Geometry check sheet. Reference: drawing and pictorial views, mm from the part's lowest x, y, z. A direction names the side the tool comes from. Give positions to 0.01 mm unless a question says otherwise; leave off trailing zeros. Loops run counter-clockwise (first coordinate to the right, second up) from the corner with the lowest first, then second, coordinate; pieces in that order, holes last. Notation, with made-up numbers: (68.25, 50.25) -> (115.25, 50.25) arc R15 cw to (115.25, 66.25) -> close; hole circle Ø8 at (48, 87). An arc over 180 degrees is marked (long way). Answer in a Markdown table with one row per item. Add a question column.
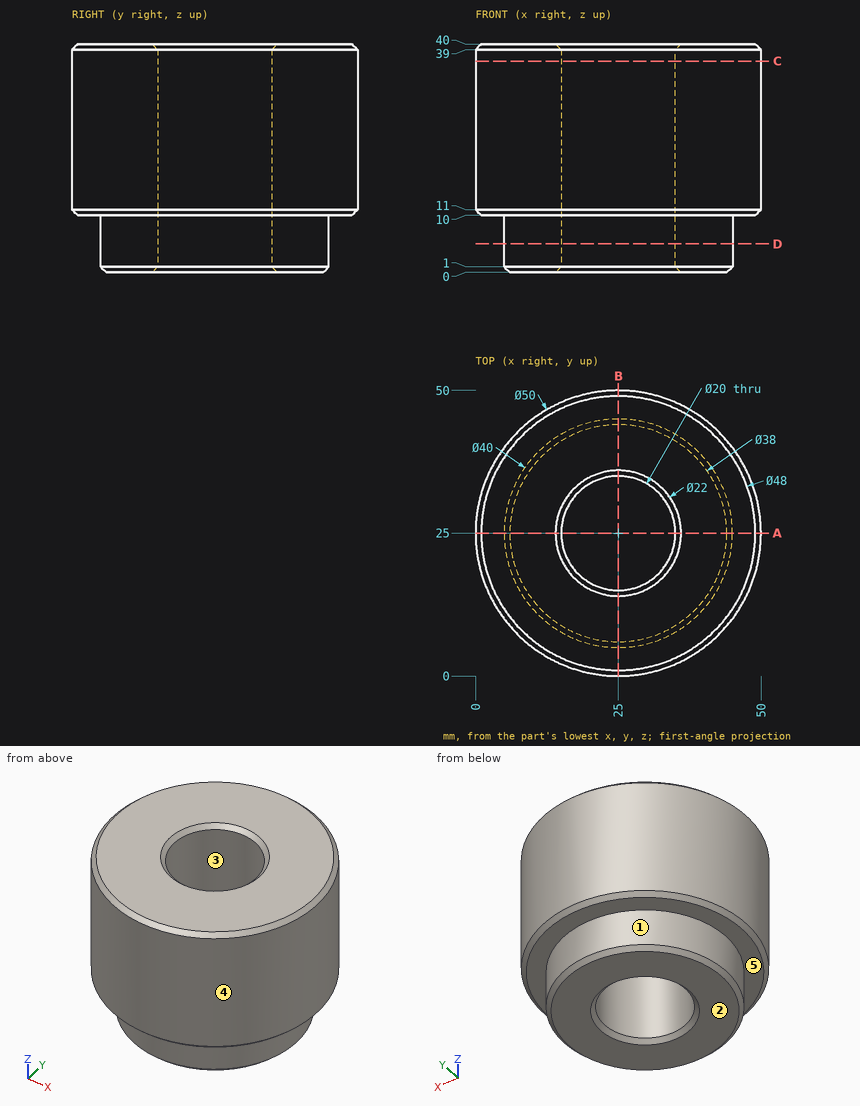
1. Release check for a two-part mould opening along Y. For the marked faces 1, 2 and 3 record: released by +Y, released by -Y, zero draft, split by the parting line, or undercut.
2. Sectioned sample at A-A (y = 25). Enter the section's corners in (x, z).
3. Sectioned sample at C-C (z = 37). Enter the section's corners in (x, y), plus the area to 3 significant figures.
4. Sectioned sample at D-D (z = 5). Enter the section's corners in (x, y), plus the area to 3 significant figures.
5. Material ranges on L1, parallel to Y at x = 25, z = 11; L2, parallel to Z at x = 42, y = 11; L3, parallel to Y at x = 17, z = 6, recorded low to high. Write a range as from..to.
6. Access from +Z, -Z, +X, -X, +Y, -Y to the whole of each face (thin tool, end or side, straight path). Record for the marked faces 4 and 5.
7. Gauge pin test, flat ends, axial feed: pin 1 Ø8 at (x, z) = (5.5, 24) entering from +Y; pin 2 Ø1.5 at (x, y) = (13.5, 42.5) entering from -Z; pin 3 Ø6 at (y, z) = (40.5, 10) entering from -X; pin 4 Ø10 at (x, y) = (27, 32) entering from +Z. Record the tip position at first contact, or that the pin passes through.
Response:
| question | item | result |
|---|---|---|
| 1 | face 1 | split by the parting line |
| 1 | face 2 | zero draft |
| 1 | face 3 | undercut |
| 2 | outline | (0, 11) -> (1, 10) -> (5, 10) -> (5, 1) -> (6, 0) -> (14, 0) -> (15, 1) -> (15, 39) -> (14, 40) -> (1, 40) -> (0, 39) -> close; (35, 1) -> (36, 0) -> (44, 0) -> (45, 1) -> (45, 10) -> (49, 10) -> (50, 11) -> (50, 39) -> (49, 40) -> (36, 40) -> (35, 39) -> close |
| 3 | outline | circle Ø50 at (25, 25); hole circle Ø20 at (25, 25) |
| 3 | area | 1,650 mm2 |
| 4 | outline | circle Ø40 at (25, 25); hole circle Ø20 at (25, 25) |
| 4 | area | 942 mm2 |
| 5 | L1 | y = 0..15, 35..50 |
| 5 | L2 | z = 10..40 |
| 5 | L3 | y = 6.67..19, 31..43.33 |
| 6 | face 4 | +Z, -Z |
| 6 | face 5 | -Z |
| 7 | pin 1 | stops at y = 44.62 |
| 7 | pin 2 | stops at z = 10 |
| 7 | pin 3 | stops at x = 3.45 |
| 7 | pin 4 | stops at z = 40 |
